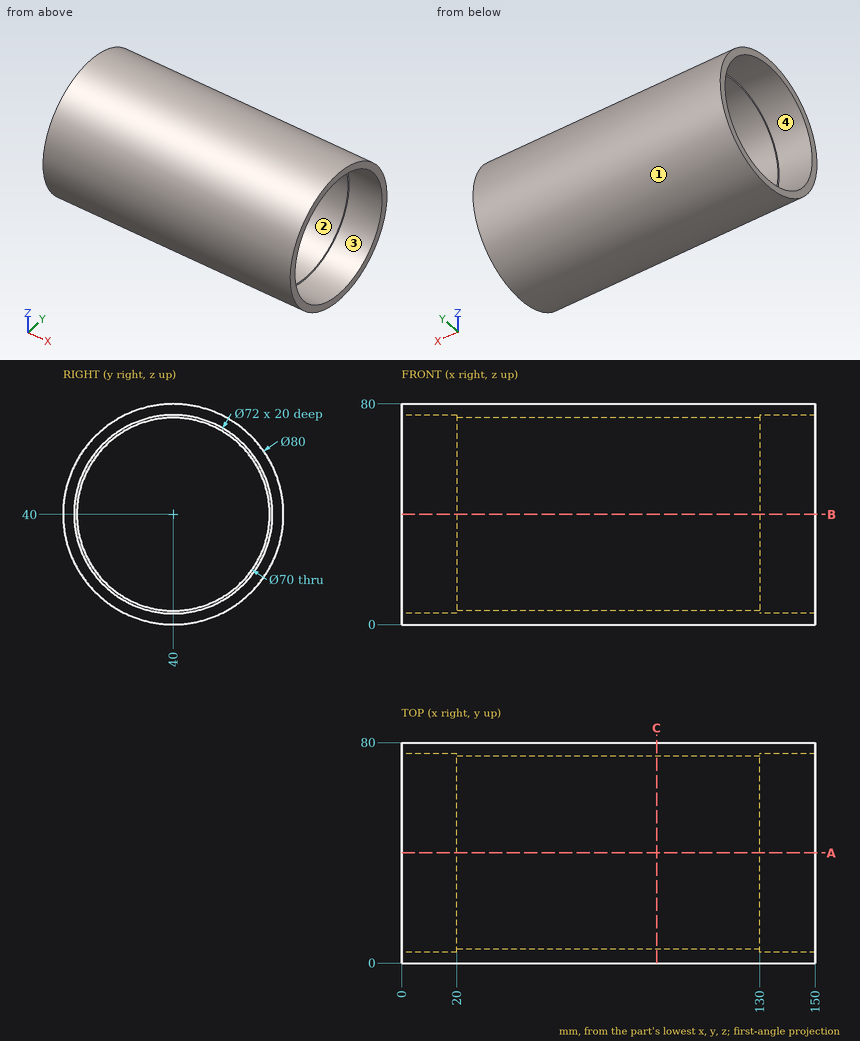
The drawing under review shows one solid part. Ordinate dimensions are in mm from its lowest x, y, z. A direction names the side the tool comes from. Coordinates: 2 decimals unless noted, no trailing zeros. Order: outer loops, then holes, each group sorted by start corner. A loop starts at its lowest first (then second) coordinate and runs counter-clockwise, first axis right, second up. Notation, with made-up numbers: (6.5, -3) -> (42.5, -3) arc R22 ccw to (42.5, 23) -> close; hole circle Ø5 at (77.5, 60.25). An arc over 180 degrees is marked (long way). One line per item, written item: value.
1) Clearance check with flat-ended pins moving along their axes: P1, Ø10, axis at x = 127.5, z = 39, coming from the +Y side; P2, Ø8, axis at x = 130, y = 67.5, coming from the -Z side; P3, Ø12, axis at y = 61, z = 24, coming from the -X side; P4, Ø8, axis at x = 96, z = 62.5, coming from the -Y side. State where each tip first meets the part, or that it passes through.
Output values:
P1: stops at y = 80
P2: stops at z = 7.63
P3: passes through
P4: stops at y = 4.54
2) To check wall thickness, follow probe 1 along Y at (x, z) = (6.75, 40); probe 2 along Y at (x, z) = (62, 40); probe 3 along Z at (x, y) = (115.5, 37). State the ranges of each line that lie inside material, in increasing order. Write a range as [from, to].
Output values:
probe 1: y = [0, 4], [76, 80]
probe 2: y = [0, 5], [75, 80]
probe 3: z = [0.11, 5.13], [74.87, 79.89]
3) Machinability: for the marked faces 3 and 4, which of the approach directions +Z, -Z, +X, -X, +Y, -Y give a long, thin tool a straight path to every point of the face, cutting with its end or side? Answer none if there is none.
Output values:
face 3: +X
face 4: -X
4) Draft analysis for pull direction Y (two halves, no side actions). For the marked faces 1 and 2, state which applies: +Y half, -Y half, draft (parallel to the pull), parting line (faces both ways), or undercut.
Output values:
face 1: parting line
face 2: undercut
5) We need section A-A, the plane y = 40. Give the boundary of the cut face in (x, z).
Output values:
outline: (0, 0) -> (150, 0) -> (150, 4) -> (130, 4) -> (130, 5) -> (20, 5) -> (20, 4) -> (0, 4) -> close; (0, 76) -> (20, 76) -> (20, 75) -> (130, 75) -> (130, 76) -> (150, 76) -> (150, 80) -> (0, 80) -> close
6) We need section C-C, the plane x = 92.5. Give the boundary of the cut face in (y, z), then the cut area to 3 significant figures.
Output values:
outline: circle Ø80 at (40, 40); hole circle Ø70 at (40, 40)
area: 1,180 mm2
